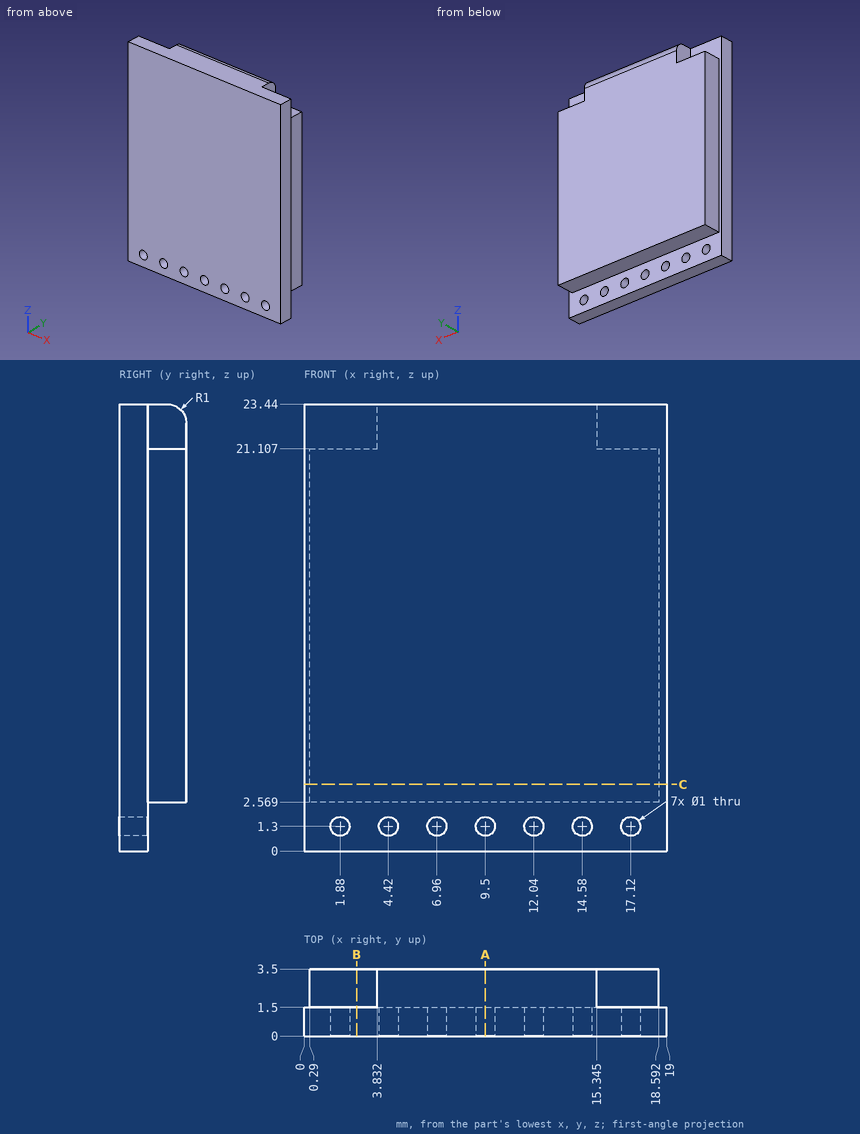
For this review, use the dimensioned drawing (mm, ordinates from the lowest corner) and the shaded views. Coordinates: 2 decimals unless noted, no trailing zeros. Write each loop counter-clockwise with the first axis right and the second up, starting at its lowest first coordinate (ties: lowest second). Pieces come first, ordered by that corner, then holes. Notation, with made-up numbers: (-36, 14) - (-22, 14) arc R23 ccw to (-22, 49) - close; hole circle Ø4 at (33, -21). An arc over 180 degrees is marked (long way). Answer in a Markdown table with one row per item. Add a question column.
Q1. Consider section B-B on x = 2.75. Give the boundary of the cut face in (y, z).
Q2. Clearance check with flat-ended pins moving along their axes: pin 1 (2 mm diameter, centred on y = 3, z = 14, fed in from +X); pin 2 (2 mm diameter, centred on y = 3, z = 18.5, fed in from -X); pin 3 (1 mm diameter, centred on x = 2.5, y = 2.5, fed in from +Z). State where each tip first meets the part, or that it passes through.
Q3. Consider section C-C on z = 3.5. Give the boundary of the cut face in (x, y), then the cut area to 3 significant figures.
Q4. To check wall thickness, follow line 1 along Z through (x, y) = (4, 2.4); line 2 along Z through (x, y) = (16.25, 1.9); line 3 along X through (y, z) = (3.35, 12.25). State the ranges of each line that lie inside material, in increasing order. Write a range as from..to.
Q5. Consider section A-A on x = 9.5. Give the boundary of the cut face in (y, z).
Answers below:
| question | item | result |
|---|---|---|
| 1 | outline | (0, 0) - (1.5, 0) - (1.5, 2.57) - (3.5, 2.57) - (3.5, 21.11) - (1.5, 21.11) - (1.5, 23.44) - (0, 23.44) - close |
| 2 | pin 1 | x = 18.59 |
| 2 | pin 2 | x = 0.29 |
| 2 | pin 3 | z = 21.11 |
| 3 | outline | (0, 0) - (19, 0) - (19, 1.5) - (18.59, 1.5) - (18.59, 3.5) - (0.29, 3.5) - (0.29, 1.5) - (0, 1.5) - close |
| 3 | area | 65.1 mm² |
| 4 | line 1 | 2.57..23.44 |
| 4 | line 2 | 2.57..21.11 |
| 4 | line 3 | 0.29..18.59 |
| 5 | outline | (0, 0) - (1.5, 0) - (1.5, 0.8) - (0, 0.8) - close; (0, 1.8) - (1.5, 1.8) - (1.5, 2.57) - (3.5, 2.57) - (3.5, 22.44) arc R1 ccw to (2.5, 23.44) - (0, 23.44) - close |
